Check sheet for the modelled part. Datum: model origin and axes. Units: mm. Face numbers are marked on the shaded views. A direction names the side the tool comes from. Round coordinates to 2 decimals unless told otherwise and drop trailing zeros. Loops run counter-clockwise (first coordinate to the right, second up) from the corner with the lowest first, then second, coordinate; pieces in that order, holes last. Notation, with made-up numbers: (69.25, 65) - (113.25, 65) arc R14 ccw to (113.25, 87) - close; hole circle Ø5 at (82, 86). An arc over 180 degrees is marked (long way). Put each result on its own line as item: value. Start each with the question number.
Item 1: Draft check along X on the marked faces 5, 6 and 7. Enter one of: pulls with the +X half, pulls with the -X half, needs draft (parallel to the pull), parting line crosses it, or undercut.
Item 2: Section check B-B, the plane y = 6.75. Record the cut outline in (x, z).
Item 3: Section check A-A, the plane x = 10. Record the cut outline in (y, z).
Item 4: Gauge pin test, flat ends, axial feed: pin 1 Ø3 at (y, z) = (2.5, 13) entering from -X; pin 2 Ø0.6 at (y, z) = (0.5, -0.5) entering from +X; pin 3 Ø0.5 at (x, z) = (21, 0) entering from -Y; pin 4 Ø4 at (x, z) = (35.6, 10.2) entering from -Y. Record the tip position at first contact, or that the pin passes through.
Item 5: Section check D-D, the plane z = 6. Record the cut outline in (x, y).
Item 6: Material ranges on line 1 along X through (y, z) = (2.85, 5); line 2 along Z through (x, y) = (14.5, 2.25); line 3 along Z through (x, y) = (-22.5, 1), recorded low to high.
Item 7: Tool access check on the marked faces 1, 2, 3 and 4. Record the directions out of +Z, -Z, +X, -X, +Y, -Y that give a thin tool (end or side, any length) a straight path to the whole face; none if there is none.
Item 8: Section check C-C, the plane x = -10. Record the cut outline in (y, z).
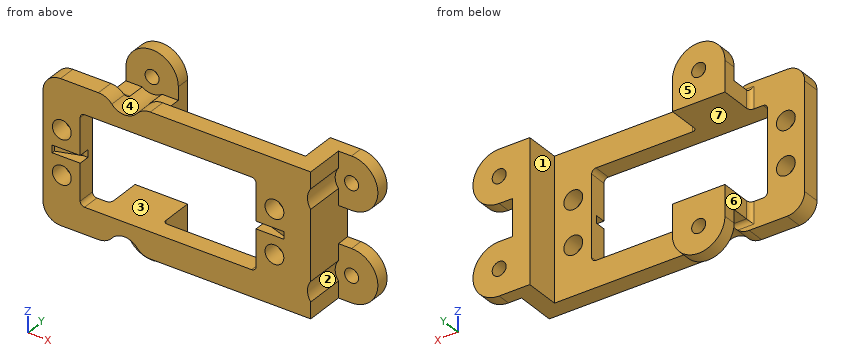
from build123d import *

# Parameters (mm, degrees)
SKETCH1_W           = 57.2
SKETCH1_H           = 32.4
SKETCH1_W_2         = 40.2
SKETCH1_H_2         = 20.4
BOSS_EXTRUDE1_DEPTH = 4
FILLET1_R           = 1
SKETCH2_R           = 2.15
CUT_EXTRUDE1_DEPTH  = 34.111931384
CUT_EXTRUDE2_DEPTH  = 0.85
SKETCH5_W           = 12
SKETCH5_H           = 4
BOSS_EXTRUDE2_DEPTH = 8
SKETCH6_R           = 1.6
BOSS_EXTRUDE3_DEPTH = 3
CUT_EXTRUDE3_REACH  = 40.732
SKETCH7_R           = 3.75
FILLET4_R           = 4
FILLET6_R           = 1
SKETCH8_W           = 4
SKETCH8_H           = 32.4
BOSS_EXTRUDE4_DEPTH = 12
SKETCH9_R           = 1.6
BOSS_EXTRUDE6_DEPTH = 3
SKETCH10_R          = 3.75
CUT_EXTRUDE4_DEPTH  = 9


with BuildPart() as part:
    # Sketch1 → Boss-Extrude1 (new body)
    with BuildSketch(Plane(origin=(0, 0, 0), x_dir=(1, 0, 0), z_dir=(0, 1, 0))):
        Rectangle(SKETCH1_W, SKETCH1_H)
        Rectangle(SKETCH1_W_2, SKETCH1_H_2, mode=Mode.SUBTRACT)
    extrude(amount=BOSS_EXTRUDE1_DEPTH)

    # Fillet1
    fillet1_edges = [part.edges().sort_by_distance(p)[0] for p in [
        (-20.1, 2, -10.2),
        (-20.1, 2, 10.2),
        (20.1, 2, 10.2),
        (20.1, 2, -10.2),
    ]]
    fillet(fillet1_edges, radius=FILLET1_R)

    # Sketch2 → Cut-Extrude1 (cut, through all)
    with BuildSketch(Plane(origin=(0, 4, 0), x_dir=(1, 0, 0), z_dir=(0, 1, 0))):
        with Locations(Location((-24.3, 5, 0), (0, 0, 270))):
            Circle(SKETCH2_R)
        with Locations(Location((-24.3, -5, 0), (0, 0, 270))):
            Circle(SKETCH2_R)
        with Locations(Location((24.3, -5, 0), (0, 0, 270))):
            Circle(SKETCH2_R)
        with Locations(Location((24.3, 5, 0), (0, 0, 270))):
            Circle(SKETCH2_R)
    extrude(amount=-CUT_EXTRUDE1_DEPTH, mode=Mode.SUBTRACT)

    # Sketch3 → Cut-Extrude2 (cut, symmetric)
    with BuildSketch(Plane.XY):
        Polygon((-26.5, 0), (-26.5, 0.7), (-21.2, 2.5), (-20.1, 2.5), (-20.1, 0), align=None)
    cut_extrude2 = extrude(amount=CUT_EXTRUDE2_DEPTH, both=True, mode=Mode.SUBTRACT)

    # Mirror1: Cut-Extrude2 across plane
    add(cut_extrude2.mirror(Plane(origin=(0, 0, 0), x_dir=(0, 0, 1), z_dir=(1, 0, 0))), mode=Mode.SUBTRACT)

    # Sketch5 → Boss-Extrude2 (add)
    with BuildSketch(Plane(origin=(0, 4, 0), x_dir=(1, 0, 0), z_dir=(0, 1, 0))):
        with Locations((-10, -12.2)):
            Rectangle(SKETCH5_W, SKETCH5_H)
    boss_extrude2 = extrude(amount=BOSS_EXTRUDE2_DEPTH)

    # Sketch6 → Boss-Extrude3 (add)
    with BuildSketch(Plane(origin=(0, 12, 0), x_dir=(1, 0, 0), z_dir=(0, 1, 0))):
        with BuildLine():
            Line((-16, -14.2), (-4, -14.2))
            Line((-4, -14.2), (-4, -17.2))
            ThreePointArc((-4, -17.2), (-10, -23.2), (-16, -17.2))
            Line((-16, -17.2), (-16, -14.2))
        make_face()
        with Locations(Location((-10, -17.2, 0), (0, 0, 270))):
            Circle(SKETCH6_R, mode=Mode.SUBTRACT)
    boss_extrude3 = extrude(amount=-BOSS_EXTRUDE3_DEPTH)

    # Cut-Extrude3: up to this face of the body (flat: up to its plane)
    cut_extrude3_end = Plane(part.part.faces().sort_by_distance((-10, 9, 23.05))[0])
    # Sketch7 → Cut-Extrude3 (cut, up to the picked face)
    with BuildSketch(Plane.XZ, mode=Mode.PRIVATE) as cut_extrude3_sk1:
        with Locations((-10, 17.2)):
            Circle(SKETCH7_R)
    cut_extrude3_tool1 = split(extrude(cut_extrude3_sk1.sketch, amount=-CUT_EXTRUDE3_REACH, mode=Mode.PRIVATE), bisect_by=cut_extrude3_end, keep=Keep.BOTH, mode=Mode.PRIVATE)
    cut_extrude3 = cut_extrude3_tool1.solids().sort_by(Axis((-10, 0, 17.2), (0, 1, 0)))[0]
    add(cut_extrude3, mode=Mode.SUBTRACT)

    # Mirror4: Boss-Extrude2, Boss-Extrude3, Cut-Extrude3 across plane
    add(boss_extrude2.mirror(Plane.XY))
    add(boss_extrude3.mirror(Plane.XY))
    add(cut_extrude3.mirror(Plane.XY), mode=Mode.SUBTRACT)

    # Fillet4
    fillet4_edges = [part.edges().sort_by_distance(p)[0] for p in [
        (-6.385791926, 2, 16.2),
        (-13.614208074, 2, 16.2),
        (-6.385791926, 2, -16.2),
        (-13.614208074, 2, -16.2),
        (-28.6, 2, -16.2),
        (-28.6, 2, 16.2),
    ]]
    fillet(fillet4_edges, radius=FILLET4_R)

    # Fillet6
    fillet6_edges = [part.edges().sort_by_distance(p)[0] for p in [
        (-14.125, 4, 14.2),
        (-16, 4, 12.2),
        (-5.875, 4, -14.2),
        (-14.125, 4, -14.2),
        (-4, 4, -12.2),
        (-16, 4, -12.2),
        (-4, 4, 12.2),
        (-5.875, 4, 14.2),
    ]]
    fillet(fillet6_edges, radius=FILLET6_R)

    # Sketch8 → Boss-Extrude4 (add)
    with BuildSketch(Plane.XZ):
        with Locations((30.6, 0)):
            Rectangle(SKETCH8_W, SKETCH8_H)
    extrude(amount=-BOSS_EXTRUDE4_DEPTH)

    # Sketch9 → Boss-Extrude6 (add)
    with BuildSketch(Plane(origin=(0, 12, 0), x_dir=(1, 0, 0), z_dir=(0, 1, 0))):
        with BuildLine():
            Line((32.6, -16.2), (32.6, -4.2))
            Line((32.6, -4.2), (35.6, -4.2))
            ThreePointArc((35.6, -4.2), (41.6, -10.2), (35.6, -16.2))
            Line((35.6, -16.2), (32.6, -16.2))
        make_face()
        with Locations(Location((35.6, -10.2, 0), (0, 0, 270))):
            Circle(SKETCH9_R, mode=Mode.SUBTRACT)
    boss_extrude6 = extrude(amount=-BOSS_EXTRUDE6_DEPTH)

    # Sketch10 → Cut-Extrude4 (cut)
    with BuildSketch(Plane.XZ):
        with Locations((35.6, 10.2)):
            Circle(SKETCH10_R)
    cut_extrude4 = extrude(amount=-CUT_EXTRUDE4_DEPTH, mode=Mode.SUBTRACT)

    # Mirror5: Boss-Extrude6, Cut-Extrude4 across plane
    add(boss_extrude6.mirror(Plane.XY))
    add(cut_extrude4.mirror(Plane.XY), mode=Mode.SUBTRACT)


solid = part.part
Check result:
1. face 5: needs draft
1. face 6: pulls with the -X half
1. face 7: undercut
2. outline: (-16, -14.2) - (-12.25, -14.2) arc R3.75 cw to (-7.75, -14.2) - (-4, -14.2) - (-4, -10.2) - (-16, -10.2) - close; (-16, 10.2) - (-4, 10.2) - (-4, 14.2) - (-7.75, 14.2) arc R3.75 cw to (-12.25, 14.2) - (-16, 14.2) - close; (28.6, -16.2) - (32.6, -16.2) - (32.6, -12.45) arc R3.75 cw to (32.6, -7.95) - (32.6, 7.95) arc R3.75 cw to (32.6, 12.45) - (32.6, 16.2) - (28.6, 16.2) - close
3. outline: (0, -16.2) - (4, -16.2) - (4, -10.2) - (0, -10.2) - close; (0, 10.2) - (4, 10.2) - (4, 16.2) - (0, 16.2) - close
4. pin 1: x = -28.6
4. pin 2: x = 32.6
4. pin 3: y = 2.48
4. pin 4: y = 9
5. outline: (-28.6, 0) - (-26.2, 0) - (-26.2, 4) - (-28.6, 4) - close; (-22.4, 0) - (-20.1, 0) - (-20.1, 4) - (-22.4, 4) - close; (20.1, 0) - (22.4, 0) - (22.4, 4) - (20.1, 4) - close; (26.2, 0) - (32.6, 0) - (32.6, 9) - (39.88, 9) - (39.88, 12) - (28.6, 12) - (28.6, 4) - (26.2, 4) - close
6. line 1: -28.6 to -26.45, -22.15 to -20.1, 20.1 to 22.15, 26.45 to 32.6
6. line 2: -16.2 to -10.2, 10.2 to 16.2
6. line 3: -16.2 to -6.18, -3.82 to -0.85, 0.85 to 3.82, 6.18 to 16.2
7. face 1: +Z, -Z, +Y
7. face 2: +X, -Y
7. face 3: +Y, -Y
7. face 4: +Z, -Y
8. outline: (0, -13.45) - (9, -13.45) - (9, -15.6) - (12, -15.6) - (12, -10.2) - (0, -10.2) - close; (0, 10.2) - (12, 10.2) - (12, 15.6) - (9, 15.6) - (9, 13.45) - (0, 13.45) - close; (9, -23.2) - (12, -23.2) - (12, -18.8) - (9, -18.8) - close; (9, 18.8) - (12, 18.8) - (12, 23.2) - (9, 23.2) - close
